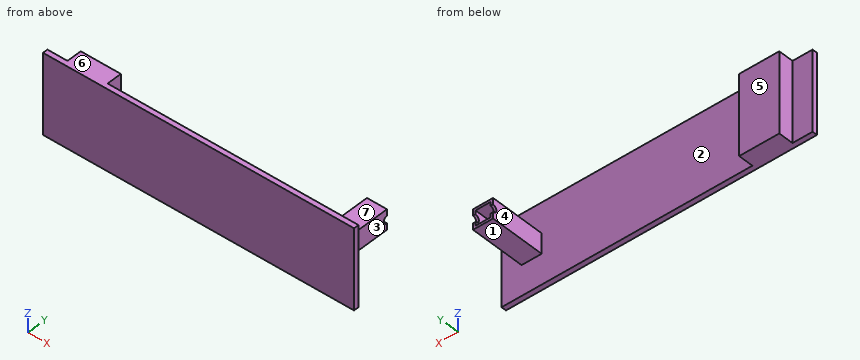
Autodesk Inventor part; units mm, degrees
ref_plane "XZ Plane" through (0, 0, 0) normal (0, 1, 0) x (-1, 0, 0)
sketch "Sketch1" plane through (0, 0, 0) normal (0, 1, 0) x (-1, 0, 0)
  line L0 (196.85, 50.8) -> (-196.85, 50.8)
  line L1 (-196.85, 50.8) -> (-196.85, -50.8)
  line L2 (-196.85, -50.8) -> (196.85, -50.8)
  line L3 (196.85, -50.8) -> (196.85, 50.8)
  line L4 (196.85, 50.8) -> (-196.85, -50.8) construction
  line L5 (-196.85, 50.8) -> (196.85, -50.8) construction
  point P0 (0, 0)
  dimension "d0" = 101.6
  dimension "d1" = 393.7
extrude "Extrusion1" add sketch "Sketch1" along normal blind 6.35
sketch "Sketch2" plane through (0, 6.35, 0) normal (0, 1, 0) x (1, 0, 0)
  line L0 (146.05, -12.7) -> (171.45, -12.7)
  line L1 (171.45, -12.7) -> (171.45, 12.7)
  line L2 (171.45, 12.7) -> (146.05, 12.7)
  line L3 (146.05, 12.7) -> (146.05, -12.7)
  line L4 (146.05, -12.7) -> (171.45, 12.7) construction
  line L5 (171.45, -12.7) -> (146.05, 12.7) construction
  line L6 (149.225, -9.525) -> (168.275, -9.525)
  line L7 (168.275, -9.525) -> (168.275, 9.525)
  line L8 (168.275, 9.525) -> (149.225, 9.525)
  line L9 (149.225, 9.525) -> (149.225, -9.525)
  line L10 (149.225, -9.525) -> (168.275, 9.525) construction
  line L11 (168.275, -9.525) -> (149.225, 9.525) construction
  line L12 (196.85, -50.8) -> (196.85, 50.8)
  line L13 (-196.85, -50.8) -> (196.85, -50.8)
  point P0 (0, 0)
  point P1 (158.75, 0)
  dimension "d4" = 25.4
  dimension "d5" = 25.4
  dimension "d6" = 3.175
  dimension "d7" = 3.175
  dimension "d8" = 25.4
  dimension "d14" = 38.1
extrude "Extrusion2" add sketch "Sketch2" along normal blind 69.7992
sketch "Sketch3" plane through (171.45, 6.35, 12.7) normal (1, 0, 0) x (0, 0, -1)
  line L0 (0, 69.7992) -> (25.4, 69.7992)
  circle A0 centre (12.7, 69.7992) radius 4.7625
  point P0 (12.7, -6.35)
  dimension "d11" = 9.525
extrude "Extrusion3" cut sketch "Sketch3" against normal through all
sketch "Sketch4" plane through (0, 6.35, 0) normal (0, 1, 0) x (1, 0, 0)
  line L0 (-171.45, -50.8) -> (-120.65, -50.8)
  line L1 (-120.65, -50.8) -> (-120.65, 50.8)
  line L2 (-120.65, 50.8) -> (-171.45, 50.8)
  line L3 (-171.45, 50.8) -> (-171.45, -50.8)
  line L4 (-171.45, -50.8) -> (-120.65, 50.8) construction
  line L5 (-120.65, -50.8) -> (-171.45, 50.8) construction
  line L6 (-196.85, 50.8) -> (-196.85, -50.8)
  line L7 (-196.85, -50.8) -> (196.85, -50.8)
  point P0 (0, 0)
  point P1 (-146.05, 0)
  dimension "d15" = 50.8
  dimension "d16" = 25.4
  dimension "d17" = 101.6
extrude "Extrusion4" add sketch "Sketch4" along normal blind 18.9992
sketch "Sketch5" plane through (0, 6.35, 0) normal (0, 1, 0) x (1, 0, 0)
  line L0 (196.85, 50.8) -> (-196.85, 50.8)
  line L1 (-101.6, 50.8) -> (101.6, 50.8)
  line L2 (101.6, 50.8) -> (101.6, 25.4)
  line L3 (101.6, 25.4) -> (-101.6, 25.4)
  line L4 (-101.6, 25.4) -> (-101.6, 50.8)
  point P0 (0, 0)
  dimension "d20" = 101.6
  dimension "d21" = 101.6
  dimension "d22" = 25.4
sketch "Sketch7" plane through (0, 6.35, 0) normal (0, 1, 0) x (1, 0, 0)
  line L0 (-196.85, -50.8) -> (196.85, -50.8)
  line L1 (-101.6, -50.8) -> (101.6, -50.8)
  line L2 (101.6, -50.8) -> (101.6, 0)
  line L3 (101.6, 0) -> (-101.6, 0)
  line L4 (-101.6, 0) -> (-101.6, -50.8)
  line L5 (-101.6, 25.4) -> (-101.6, 50.8)
  line L6 (101.6, 50.8) -> (101.6, 25.4)
  line L7 (101.6, 25.4) -> (-101.6, 25.4)
  point P0 (0, 0)
  dimension "d28" = 25.4
equation "\"d0\" = width"
equation "\"d1\" = length"
equation "\"d2\" = thickness"
equation "\"width\" = 101.6"
equation "\"length\" = 393.7"
equation "\"thickness\" = 6.35"
properties part number "SupportPlateToAttachToRobotBase" material "Aluminum 6061"
The model under review builds one solid part; all positions refer to its coordinate system, in mm. Face numbers are marked on the shaded views. A direction names the side the tool comes from. Round coordinates to 2 decimals unless told otherwise and drop trailing zeros. Write each loop counter-clockwise with the first axis right and the second up, starting at its lowest first coordinate (ties: lowest second). Pieces come first, ordered by that corner, then holes. Notation, with made-up numbers: (-38, 39) -> (-32, 39) arc R21 cw to (-32, 53) -> close; hole circle Ø1 at (34.25, 41). An arc over 180 degrees is marked (long way). Answer as a JSON object with one key per item and string values.
1. To check wall thickness, follow line 1 along X through (y, z) = (54, -5.5) (3 decimals); line 2 along X through (y, z) = (11.5, 8.5) (3 decimals); line 3 along Z through (x, y) = (162, 49.5) (3 decimals). State the ranges of each line that lie inside material, in increasing order.
Results found:
{"line 1": "x = 146.05 to 149.225, 168.275 to 171.45", "line 2": "x = -171.45 to -120.65, 146.05 to 149.225, 168.275 to 171.45", "line 3": "z = -12.7 to -9.525, 9.525 to 12.7"}
2. Machinability: for the marked faces 5, 6 and 7, which of the approach directions +Z, -Z, +X, -X, +Y, -Y give a long, thin tool a straight path to every point of the face, cutting with its end or side? Answer none if there is none.
Results found:
{"face 5": "+Z, -Z, -X, +Y", "face 6": "+Z, +X, -X, +Y, -Y", "face 7": "+Z, +X, +Y"}
3. We need section C-C on z = -28. State the section outline as (x, y) points.
Results found:
{"outline": "(-196.85, 0) -> (196.85, 0) -> (196.85, 6.35) -> (-120.65, 6.35) -> (-120.65, 25.35) -> (-171.45, 25.35) -> (-171.45, 6.35) -> (-196.85, 6.35) -> close"}
4. The part is to be moulded in two halves that separate along X. For the marked faces 1, 2, 3 and 4, say which applies: pulls with the +X half, pulls with the -X half, needs draft (parallel to the pull), parting line crosses it, or undercut.
Results found:
{"face 1": "needs draft", "face 2": "undercut", "face 3": "pulls with the +X half", "face 4": "undercut"}
5. We need section A-A on y = 12. State the section outline as (x, z) points (3 decimals), and give its area (3 significant figures).
Results found:
{"outline": "(-171.45, -50.8) -> (-120.65, -50.8) -> (-120.65, 50.8) -> (-171.45, 50.8) -> close; (146.05, -12.7) -> (171.45, -12.7) -> (171.45, 12.7) -> (146.05, 12.7) -> close; hole (149.225, -9.525) -> (168.275, -9.525) -> (168.275, 9.525) -> (149.225, 9.525) -> close", "area": "5,440 mm^2"}
6. Clearance check with flat-ended pins moving along their axes: pin 1 (5.5 mm diameter, centred on x = 157.5, y = 55, fed in from -Z); pin 2 (20.5 mm diameter, centred on x = 155, y = 26.5, fed in from +Z); pin 3 (6 mm diameter, centred on x = -16.5, z = 9.5, fed in from +Y); pin 4 (21 mm diameter, centred on y = 13, z = 11.5, fed in from -X). State where each tip first meets the part, or that it passes through.
Results found:
{"pin 1": "stops at z = -12.7", "pin 2": "stops at z = 12.7", "pin 3": "stops at y = 6.35", "pin 4": "stops at x = -196.85"}
7. We need section B-B on y = 55.5. State the section outline as (x, z) points (3 decimals).
Results found:
{"outline": "(146.05, -12.7) -> (171.45, -12.7) -> (171.45, 12.7) -> (146.05, 12.7) -> close; hole (149.225, -9.525) -> (168.275, -9.525) -> (168.275, 9.525) -> (149.225, 9.525) -> close"}
8. We need section D-D on z = 0. State the section outline as (x, y) points (3 decimals), and give its area (3 significant figures).
Results found:
{"outline": "(-196.85, 0) -> (196.85, 0) -> (196.85, 6.35) -> (171.45, 6.35) -> (171.45, 71.387) -> (168.275, 71.387) -> (168.275, 6.35) -> (149.225, 6.35) -> (149.225, 71.387) -> (146.05, 71.387) -> (146.05, 6.35) -> (-120.65, 6.35) -> (-120.65, 25.349) -> (-171.45, 25.349) -> (-171.45, 6.35) -> (-196.85, 6.35) -> close", "area": "3,880 mm^2"}
